```python
from build123d import *

# Parameters (mm, degrees)
SKETCH1_W            = 6.35
SKETCH1_H            = 6.35
BOSS_EXTRUDE1_DEPTH  = 4.7625
SKETCH3_R            = 1.5875
BOSS_EXTRUDE2_DEPTH  = 1.5875
BOSS_EXTRUDE3_START  = -1.5875
SKETCH4_R            = 1.5875
BOSS_EXTRUDE3_DEPTH  = 1.5875
SKETCH5_R            = 1.190625
BOSS_EXTRUDE4_START  = -8.89
SKETCH7_R            = 1.74625
BOSS_EXTRUDE4_DEPTH  = 9.68375
SKETCH8_R            = 2.38125
BOSS_EXTRUDE5_DEPTH  = 0.79375
FILLET2_R            = 0.254
FILLET3_R            = 0.254
FILLET4_R            = 0.254
FILLET2_OF_MIRROR3_R = 0.254
FILLET3_OF_MIRROR3_R = 0.254
FILLET4_OF_MIRROR3_R = 0.254
SKETCH9_W            = 52.511518924
SKETCH9_H            = 9.759118081
CUT_EXTRUDE1_DEPTH   = 27.610644864


with BuildPart() as part:
    # Sketch1 → Boss-Extrude1 (new body)
    with BuildSketch(Plane.XY):
        with Locations((1.55575, 0.635)):
            Rectangle(SKETCH1_W, SKETCH1_H)
    extrude(amount=BOSS_EXTRUDE1_DEPTH)

    # Sketch3 → Boss-Extrude2 (add)
    with BuildSketch(Plane(origin=(4.73075, 0, 0), x_dir=(0, 0, -1), z_dir=(1, 0, 0))):
        with Locations((-7.9375, 0.635)):
            Circle(SKETCH3_R)
        with BuildLine():
            Line((-4.7625, -2.54), (-4.7625, 3.81))
            Line((-4.7625, 3.81), (-8.590657552, 2.081907552))
            ThreePointArc((-8.590657552, 2.081907552), (-7.076318069, 1.968612362), (-6.35, 0.635))
            ThreePointArc((-6.35, 0.635), (-7.076318069, -0.698612362), (-8.590657552, -0.811907552))
            Line((-8.590657552, -0.811907552), (-4.7625, -2.54))
        make_face()
    extrude(amount=-BOSS_EXTRUDE2_DEPTH)

    # Sketch4 → Boss-Extrude3 (add)
    with BuildSketch(Plane.ZY.offset(1.61925).offset(BOSS_EXTRUDE3_START)):
        with BuildLine():
            Line((4.7625, -2.54), (8.590657552, -0.811907552))
            ThreePointArc((8.590657552, -0.811907552), (6.35, 0.635), (8.590657552, 2.081907552))
            Line((8.590657552, 2.081907552), (4.7625, 3.81))
            Line((4.7625, 3.81), (4.7625, -2.54))
        make_face()
        with Locations((7.9375, 0.635)):
            Circle(SKETCH4_R)
    extrude(amount=BOSS_EXTRUDE3_DEPTH)

    # Sweep1: sweep along a path in Sketch6
    with BuildLine(Plane.XY.offset(7.9375)) as sweep1_path:
        Line((-1.61925, 0.635), (4.73075, 0.635))
        Line((4.73075, 0.635), (13.225286858, 0.635))
        ThreePointArc((13.225286858, 0.635), (14.242444101, 0.553005356), (15.233333172, 0.309138943))
        Line((15.233333172, 0.309138943), (23.78075, -2.54))
    # Sketch5 → Sweep1 (sweep)
    with BuildSketch(Plane.ZY.offset(1.61925)):
        with Locations((7.9375, 0.635)):
            Circle(SKETCH5_R)
    sweep1 = sweep(path=sweep1_path.line)

    # Mirror1: Sweep1 across plane
    add(sweep1.mirror(Plane.ZY.offset(-1.55575)))

    # Sketch7 → Boss-Extrude4 (add)
    with BuildSketch(Plane(origin=(22.164675, -7.388225, 0), x_dir=(0, 0, -1), z_dir=(0.9486832980505139, -0.31622776601683794, 0)).offset(BOSS_EXTRUDE4_START)):
        with Locations(Location((-7.9375, 5.11047787, 0), (0, 0, 90))):
            Circle(SKETCH7_R)
    boss_extrude4 = extrude(amount=BOSS_EXTRUDE4_DEPTH)

    # Sketch8 → Boss-Extrude5 (add)
    with BuildSketch(Plane(origin=(13.73088048, -4.57696016, 0), x_dir=(0, 0, 1), z_dir=(-0.9486832980505139, 0.316227766016838, 0))):
        with Locations(Location((7.9375, 5.11047787, 0), (0, 0, 90))):
            Circle(SKETCH8_R)
    boss_extrude5 = extrude(amount=BOSS_EXTRUDE5_DEPTH)

    # Fillet2
    fillet2_edges = [part.edges().sort_by_distance(p)[0] for p in [
        (23.981554631, -4.447643999, 7.9375),
    ]]
    fillet(fillet2_edges, radius=FILLET2_R)

    # Fillet3
    fillet3_edges = [part.edges().sort_by_distance(p)[0] for p in [
        (14.794742744, -1.385373369, 7.9375),
    ]]
    fillet(fillet3_edges, radius=FILLET3_R)

    # Fillet4
    fillet4_edges = [part.edges().sort_by_distance(p)[0] for p in [
        (13.840920745, -1.736781474, 7.9375),
        (14.593938113, -1.987787264, 7.9375),
    ]]
    fillet(fillet4_edges, radius=FILLET4_R)

    # Mirror3: Boss-Extrude4, Boss-Extrude5 across plane
    add(boss_extrude4.mirror(Plane.ZY.offset(-1.55575)))
    add(boss_extrude5.mirror(Plane.ZY.offset(-1.55575)))

    # Fillet2 of Mirror3
    fillet2_of_mirror3_edges = [part.edges().sort_by_distance(p)[0] for p in [
        (-20.870054631, -4.447643999, 7.9375),
    ]]
    fillet(fillet2_of_mirror3_edges, radius=FILLET2_OF_MIRROR3_R)

    # Fillet3 of Mirror3
    fillet3_of_mirror3_edges = [part.edges().sort_by_distance(p)[0] for p in [
        (-11.683242744, -1.385373369, 7.9375),
    ]]
    fillet(fillet3_of_mirror3_edges, radius=FILLET3_OF_MIRROR3_R)

    # Fillet4 of Mirror3
    fillet4_of_mirror3_edges = [part.edges().sort_by_distance(p)[0] for p in [
        (-10.729420745, -1.736781474, 7.9375),
        (-11.482438113, -1.987787264, 7.9375),
    ]]
    fillet(fillet4_of_mirror3_edges, radius=FILLET4_OF_MIRROR3_R)

    # Sketch9 → Cut-Extrude1 (cut, through all)
    with BuildSketch(Plane.XY.offset(7.9375)):
        with Locations((1.780183147, -0.320056159)):
            Rectangle(SKETCH9_W, SKETCH9_H)
    extrude(amount=-CUT_EXTRUDE1_DEPTH, mode=Mode.SUBTRACT)


solid = part.part
```
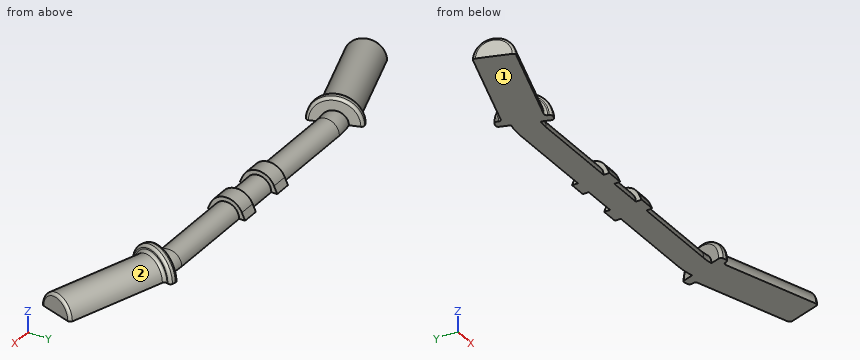
Model file for the job. Use its own axes, mm. Face numbers are marked on the shaded views. Coordinates: 2 decimals unless noted, no trailing zeros. Order: outer loops, then holes, each group sorted by start corner. A loop starts at its lowest first (then second) coordinate and runs counter-clockwise, first axis right, second up. Notation, with made-up numbers: (70.5, 62) -> (75.5, 62) arc R14 cw to (75.5, 84) -> close; hole circle Ø11 at (25.25, 80). An arc over 180 degrees is marked (long way). Return JSON: item names as keys, results as strings.
Item 1: Slice it at B-B (x = -6). Write the cut outline in (y, z) (1 decimal), then the cut area to 3 significant figures.
Model answer:
{"outline": "(-0.6, 7.9) -> (1.8, 7.9) arc R1.2 ccw to start", "area": "2.23 mm²"}
Item 2: Pin check, flat tip, straight feed: P1, Ø1.5, axis at x = 0, y = -1.5, coming from the +Z side. Stop position of the tip, or through.
Model answer:
{"P1": "stops at z = 8.71"}
Item 3: Slice it at A-A (x = 4). Write the cut outline in (y, z) (1 decimal), then the cut area to 3 significant figures.
Model answer:
{"outline": "(-1.1, 7.9) -> (2.4, 7.9) -> (2.1, 8.6) arc R1.6 ccw to (-0.8, 8.6) -> close", "area": "4.03 mm²"}
Item 4: Mould opens along X. For the marked faces 1 and 2 say: pulls with the +X half, pulls with the -X half, needs draft (parallel to the pull), parting line crosses it, or undercut.
Model answer:
{"face 1": "needs draft", "face 2": "undercut"}
Item 5: Wall check: line 1 along X through (y, z) = (1.5, 9.2); line 2 along X through (y, z) = (2, 8.15); line 3 along X through (y, z) = (1.75, 9.25). Give the ranges that are in metal, low to high. Write a range as from..to.
Model answer:
{"line 1": "x = -12.72..-11.81, -1.62..-0.03, 3.14..4.73, 14.92..15.83", "line 2": "x = -12.86..-11.98, -1.62..-0.03, 3.14..4.73, 15.09..15.97", "line 3": "x = -12.73..-11.89, 15..15.84"}
